For this review, take the finished solid that the model builds, in its own axes (mm). Face numbers are marked on the shaded views. A direction names the side the tool comes from. Round coordinates to 2 decimals unless told otherwise and drop trailing zeros. Order: outer loops, then holes, each group sorted by start corner. A loop starts at its lowest first (then second) coordinate and runs counter-clockwise, first axis right, second up. Notation, with made-up numbers: (43.25, 18.25) -> (58.25, 18.25) arc R19 cw to (58.25, 43.25) -> close; hole circle Ø4 at (-31, -7). An arc over 180 degrees is marked (long way). Use a Markdown table: item, result. Add a question column.
1) Consider section B-B (y = 1). State the section outline as (x, z) points, plus the area to 3 significant figures.
2) Draft analysis for pull direction X (two halves, no side actions). For the marked faces 1, 2 and 3, state which applies: pulls with the +X half, pulls with the -X half, needs draft (parallel to the pull), parting line crosses it, or undercut.
3) Wall thickness on line 1 along Z through (x, y) = (-11, 4.75); line 2 along Z through (x, y) = (-6, 5.5); line 3 along Z through (x, y) = (16, 6.25): over which ranges is each line inside the solid? List them lowest first. Write a range as [from, to].
4) Clearance check with flat-ended pins moving along their axes: P1, Ø2.5, axis at y = 4, z = -12, coming from the -X side; P2, Ø1, axis at y = 5, z = 4.5, coming from the +X side; P3, Ø1.2, axis at y = 4, z = 11, coming from the -X side; P4, Ø1.6, axis at x = -12.12, z = -0.12, coming from the -Y side (3 decimals). State where each tip first meets the part, or that it passes through.
5) Machinability: for the marked faces 4, 5 and 6, which of the approach directions +Z, -Z, +X, -X, +Y, -Y give a long, thin tool a straight path to every point of the face, cutting with its end or side? Answer none if there is none.
6) Consider section A-A (y = 4). Give the number of separate pieces and of enclosed holes in the cut face, plus the area to 3 significant figures.
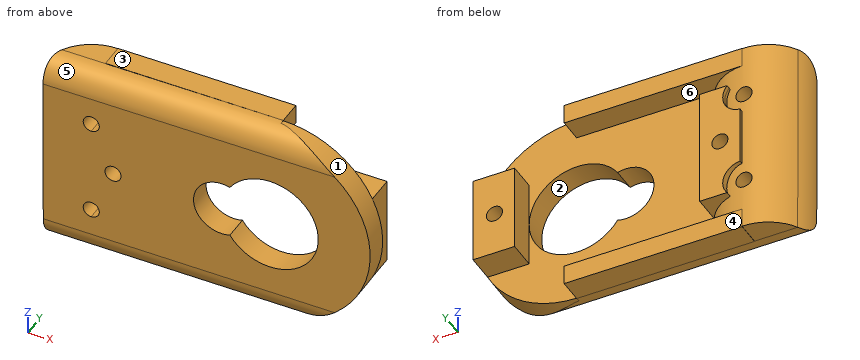
```python
from build123d import *

# Parameters (mm, degrees)
CROQUIS1_R              = 1.00000007
CROQUIS1_R_2            = 1.000000043
CROQUIS1_R_3            = 0.999999659
SALIENTE_EXTRUIR1_DEPTH = 3
SALIENTE_EXTRUIR2_REACH = 34.647
CROQUIS3_W              = 22.095085155
CROQUIS3_H              = 2.45
CROQUIS3_W_2            = 5.163600355
CROQUIS3_H_2            = 11
CROQUIS3_R              = 1
SALIENTE_EXTRUIR3_DEPTH = 3
CROQUIS4_W              = 5.163600355
CROQUIS4_H              = 11
CROQUIS4_R              = 1
SALIENTE_EXTRUIR4_DEPTH = 0.5
CORTAR_EXTRUIR1_DEPTH   = 30.5
CROQUIS6_R              = 1.000000043
CROQUIS6_R_2            = 1.00000007
CROQUIS6_R_3            = 0.999999659
CORTAR_EXTRUIR2_DEPTH   = 30.5
REDONDEO1_R             = 3


with BuildPart() as part:
    # Croquis1 → Saliente-Extruir1 (new body)
    with BuildSketch(Plane(origin=(0, 0, 0), x_dir=(1, 0, 0), z_dir=(0, 1, 0))):
        with BuildLine():
            Line((-20.817493094, 12.573865304), (7.482507574, 12.623865495))
            Line((7.482507574, 12.623865495), (7.482507574, 12.573916185))
            ThreePointArc((7.482507574, 12.573916185), (19.826569133, 0.122006117), (7.482507574, -12.329903951))
            Line((7.482507574, -12.329903951), (7.482507574, -12.376134505))
            Line((7.482507574, -12.376134505), (-20.817493094, -12.326134314))
            Line((-20.817493094, -12.326134314), (-20.817493094, 12.573865304))
        make_face()
        with Locations(Location((-12.11749246, 0.123865663, 0), (0, 0, 270))):
            Circle(CROQUIS1_R, mode=Mode.SUBTRACT)
        with Locations(Location((-14.817492891, 6.123865452, 0), (0, 0, 270))):
            Circle(CROQUIS1_R_2, mode=Mode.SUBTRACT)
        with Locations(Location((-14.817492524, -5.876134505, 0), (0, 0, 270))):
            Circle(CROQUIS1_R_3, mode=Mode.SUBTRACT)
        with BuildLine():
            ThreePointArc((2.403340998, -3.223954765), (13.382507625, 0.123866695), (2.403340083, 3.471685154))
            ThreePointArc((2.403340083, 3.471685154), (-2.117492981, 0.123864576), (2.403340998, -3.223954765))
        make_face(mode=Mode.SUBTRACT)
    extrude(amount=SALIENTE_EXTRUIR1_DEPTH)

    # Saliente-Extruir2: up to this plane
    saliente_extruir2_end = Plane(origin=(-20.817493094, 3, -12.573865304), z_dir=(0.001766788392819182, 0, 0.9999984392281696))
    # Croquis2 → Saliente-Extruir2 (add, up to the surface)
    with BuildSketch(Plane(origin=(-0.02184262, 0, 12.362875885), x_dir=(0.9999984392281696, 0, 0.001766788392856574), z_dir=(-0.001766788392856574, 0, 0.9999984392281696)), mode=Mode.PRIVATE) as saliente_extruir2_sk1:
        with BuildLine():
            Line((-9.599530509, 3), (-19.991835354, 3))
            ThreePointArc((-19.991835354, 3), (-14.795682931, 6), (-9.599530509, 3))
        make_face()
    saliente_extruir2_tool1 = split(extrude(saliente_extruir2_sk1.sketch, amount=-SALIENTE_EXTRUIR2_REACH, mode=Mode.PRIVATE), bisect_by=saliente_extruir2_end, keep=Keep.BOTH, mode=Mode.PRIVATE)
    add(saliente_extruir2_tool1.solids().sort_by_distance((-14.817502, 4.230121, 12.336735))[0])

    # Croquis3 → Saliente-Extruir3 (add)
    # profile 1 of 4: a face of its own
    with BuildSketch(Plane(origin=(0, 3, 0), x_dir=(1, 0, 0), z_dir=(0, 1, 0))):
        with Locations((-3.565035003, -11.151134505)):
            Rectangle(CROQUIS3_W, CROQUIS3_H)
    # profile 2 of 4: a face of its own
    with BuildSketch(Plane(origin=(0, 3, 0), x_dir=(1, 0, 0), z_dir=(0, 1, 0))):
        with Locations((-3.565035003, 11.398865495)):
            Rectangle(CROQUIS3_W, CROQUIS3_H)
    # profile 3 of 4: a face of its own
    with BuildSketch(Plane(origin=(0, 3, 0), x_dir=(1, 0, 0), z_dir=(0, 1, 0))):
        with BuildLine():
            Line((-13.012577984, 7.623865495), (-9.612577581, 7.623865495))
            Line((-9.612577581, 7.623865495), (-9.612577581, -7.376134505))
            Line((-9.612577581, -7.376134505), (-13.012577581, -7.376134505))
            ThreePointArc((-13.012577581, -7.376134505), (-12.651343128, -4.973075952), (-14.612577581, -3.538244886))
            Line((-14.612577581, -3.538244886), (-14.612577581, 3.785975877))
            ThreePointArc((-14.612577581, 3.785975877), (-12.651343414, 5.220807096), (-13.012577984, 7.623865495))
        make_face()
    # profile 4 of 4: a face of its own
    with BuildSketch(Plane(origin=(0, 3, 0), x_dir=(1, 0, 0), z_dir=(0, 1, 0))):
        with Locations((15.964307803, 0.122006117)):
            Rectangle(CROQUIS3_W_2, CROQUIS3_H_2)
        with Locations(Location((15.884187935, 0.123865875, 0), (0, 0, 270))):
            Circle(CROQUIS3_R, mode=Mode.SUBTRACT)
    extrude(amount=SALIENTE_EXTRUIR3_DEPTH)

    # Croquis4 → Saliente-Extruir4 (add)
    # profile 1 of 2: a face of its own
    with BuildSketch(Plane(origin=(0, 6, 0), x_dir=(1, 0, 0), z_dir=(0, 1, 0))):
        with Locations((15.964307803, 0.122006117)):
            Rectangle(CROQUIS4_W, CROQUIS4_H)
        with Locations(Location((15.884187935, 0.123865875, 0), (0, 0, 270))):
            Circle(CROQUIS4_R, mode=Mode.SUBTRACT)
    # profile 2 of 2: a face of its own
    with BuildSketch(Plane(origin=(0, 6, 0), x_dir=(1, 0, 0), z_dir=(0, 1, 0))):
        with BuildLine():
            Line((-13.012577576, -7.376134508), (-9.612577581, -7.376134505))
            Line((-9.612577581, -7.376134505), (-9.612577581, 7.623865495))
            Line((-9.612577581, 7.623865495), (-13.012577984, 7.623865495))
            ThreePointArc((-13.012577984, 7.623865495), (-12.651343414, 5.220807096), (-14.612577581, 3.785975877))
            Line((-14.612577581, 3.785975877), (-14.612577581, -3.538244892))
            ThreePointArc((-14.612577581, -3.538244892), (-12.651343124, -4.97307595), (-13.012577576, -7.376134508))
        make_face()
    extrude(amount=SALIENTE_EXTRUIR4_DEPTH)

    # Croquis5 → Cortar-Extruir1 (cut)
    with BuildSketch(Plane(origin=(-0.02184262, 0, 12.362875885), x_dir=(0.9999984392281696, 0, 0.001766788392856574), z_dir=(-0.001766788392856574, 0, 0.9999984392281696))):
        with BuildLine():
            ThreePointArc((-19.991835354, 3), (-17.725768159, 5.235895392), (-14.634858473, 5.997844237))
            Line((-14.634858473, 5.997844237), (-14.634858473, 8.229597487))
            ThreePointArc((-14.634858473, 8.229597487), (-20.558857666, 5.876900228), (-23.026851701, 0))
            Line((-23.026851701, 0), (-20.795682931, 0))
            Line((-20.795682931, 0), (-20.795682931, 3))
            Line((-20.795682931, 3), (-19.991835354, 3))
        make_face()
        with BuildLine():
            ThreePointArc((-20.795682931, 0), (-20.591237889, 1.552914271), (-19.991835354, 3))
            Line((-19.991835354, 3), (-20.795682931, 3))
            Line((-20.795682931, 3), (-20.795682931, 0))
        make_face()
    extrude(amount=-CORTAR_EXTRUIR1_DEPTH, mode=Mode.SUBTRACT)

    # Croquis6 → Cortar-Extruir2 (cut)
    with BuildSketch(Plane.XZ):
        with Locations(Location((-14.817492891, -6.123865452, 0), (0, 0, 270))):
            Circle(CROQUIS6_R)
        with Locations(Location((-12.11749246, -0.123865663, 0), (0, 0, 90))):
            Circle(CROQUIS6_R_2)
        with Locations(Location((-14.817492524, 5.876134505, 0), (0, 0, 270))):
            Circle(CROQUIS6_R_3)
    extrude(amount=-CORTAR_EXTRUIR2_DEPTH, mode=Mode.SUBTRACT)

    # Redondeo1
    redondeo1_edges = [part.edges().sort_by_distance(p)[0] for p in [
        (-6.645496142, 0, -12.598904263),
        (-6.66749276, 0, 12.35113441),
    ]]
    fillet(redondeo1_edges, radius=REDONDEO1_R - 0.0001)  # a hair under: the kernel refuses the full size


solid = part.part
```
Results list:
| question | item | result |
|---|---|---|
| 1 | outline | (-20.73, 11.56) -> (-20.69, -11.81) -> (11.51, -11.87) arc R12.45 ccw to (11.52, 11.62) -> close; hole circle Ø2 at (-14.82, -6.12); hole circle Ø2 at (-14.82, 5.88); hole circle Ø2 at (-12.12, -0.12); hole (2.4, -3.47) arc R6 ccw (long way) to (2.4, 3.22) arc R3.5 ccw (long way) to start |
| 1 | area | 753 mm2 |
| 2 | face 1 | pulls with the +X half |
| 2 | face 2 | undercut |
| 2 | face 3 | needs draft |
| 3 | line 1 | [-12.62, -10.17], [-7.62, 7.38], [9.93, 12.38] |
| 3 | line 2 | [-12.62, -10.17], [9.93, 12.38] |
| 3 | line 3 | [-5.62, -1.12], [0.87, 5.38] |
| 4 | P1 | x = -20.11 |
| 4 | P2 | x = 18.55 |
| 4 | P3 | x = -19.76 |
| 4 | P4 | through |
| 5 | face 4 | -Z, +X, -X, +Y |
| 5 | face 5 | +Z, -X, -Y |
| 5 | face 6 | +X, +Y |
| 6 | separate pieces | 2 |
| 6 | enclosed holes | 4 |
| 6 | area | 365 mm2 |
